The model under review builds one solid part; all positions refer to its coordinate system, in mm. A direction names the side the tool comes from. Round coordinates to 2 decimals unless told otherwise and drop trailing zeros. Order: outer loops, then holes, each group sorted by start corner. A loop starts at its lowest first (then second) coordinate and runs counter-clockwise, first axis right, second up.
```python
from build123d import *

# Parameters (mm, degrees)
SKETCH_1_W          = 50
SKETCH_1_H          = 35
EXTRUDE_1_DEPTH     = 109
SKETCH_2_W          = 50
SKETCH_2_H          = 25
CUT_EXTRUDE_1_DEPTH = 99
CUT_EXTRUDE_2_DEPTH = 11


with BuildPart() as part:
    # 草图1 → 凸台-拉伸1 (new body)
    with BuildSketch(Plane(origin=(0, 0, 0), x_dir=(1, 0, 0), z_dir=(0, 1, 0))):
        Rectangle(SKETCH_1_W, SKETCH_1_H)
    extrude(amount=EXTRUDE_1_DEPTH)

    # 草图2 → 切除-拉伸1 (cut)
    with BuildSketch(Plane(origin=(0, 109, 0), x_dir=(1, 0, 0), z_dir=(0, 1, 0))):
        with Locations((0, 5)):
            Rectangle(SKETCH_2_W, SKETCH_2_H)
    extrude(amount=-CUT_EXTRUDE_1_DEPTH, mode=Mode.SUBTRACT)

    # 草图3 → 切除-拉伸2 (cut, through all)
    with BuildSketch(Plane(origin=(0, 10, 0), x_dir=(1, 0, 0), z_dir=(0, 1, 0))):
        with BuildLine():
            Line((-20.7, 1.5), (-20.7, 9.5))
            ThreePointArc((-20.7, 9.5), (-17.5, 12.7), (-14.3, 9.5))
            Line((-14.3, 9.5), (-14.3, 1.5))
            ThreePointArc((-14.3, 1.5), (-17.5, -1.7), (-20.7, 1.5))
        make_face()
        with BuildLine():
            Line((20.7, 1.5), (20.7, 9.5))
            ThreePointArc((20.7, 9.5), (17.5, 12.7), (14.3, 9.5))
            Line((14.3, 9.5), (14.3, 1.5))
            ThreePointArc((14.3, 1.5), (17.5, -1.7), (20.7, 1.5))
        make_face()
    extrude(amount=-CUT_EXTRUDE_2_DEPTH, mode=Mode.SUBTRACT)


solid = part.part
```
(1) To check wall thickness, follow probe 1 along Z at (x, y) = (-18, 100); probe 2 along Y at (x, z) = (20, 7). State the ranges of each line that lie inside material, in increasing order.
Data:
probe 1: z = 7.5 to 17.5
probe 2: y = 0 to 10
(2) Consider section C-C (x = 6). Write out the cut boundary in (y, z), and give its area (3 significant figures).
Data:
outline: (0, -17.5) - (10, -17.5) - (10, 7.5) - (109, 7.5) - (109, 17.5) - (0, 17.5) - close
area: 1,340 mm2
(3) Consider section A-A (z = -8.5). Write out the cut boundary in (x, y), and give its area (3 significant figures).
Data:
outline: (-25, 0) - (-20.7, 0) - (-20.7, 10) - (-25, 10) - close; (-14.3, 0) - (14.3, 0) - (14.3, 10) - (-14.3, 10) - close; (20.7, 0) - (25, 0) - (25, 10) - (20.7, 10) - close
area: 372 mm2
(4) Consider section D-D (y = 102). Write out the cut boundary in (x, z), and give its area (3 significant figures).
Data:
outline: (-25, 7.5) - (25, 7.5) - (25, 17.5) - (-25, 17.5) - close
area: 500 mm2
(5) For faces 1 (the flat face through (0, 5, -17.5)), 2 (the flat face through (0, 10, -5)), 3 (the flat face through (-20.7, 5, -5)), list the 3-axis set-ups (+Z, -Z, +X, -X, +Y, -Y) from which the entire face can be reached by the end or side of a thin tool; tool diameter is ignored.
Data:
face 1: -Z, +X, -X, +Y, -Y
face 2: -Z, +X, -X, +Y
face 3: +Y, -Y
(6) Draft analysis for pull direction Z (two halves, no side actions). For faces 4 (the flat face through (14.3, 5, -6)), 5 (the flat face through (0, 60, 7.5)), 6 (the flat face through (25, 42, 8)), state which applies: pulls with the +Z half, pulls with the -Z half, needs draft (parallel to the pull), parting line crosses it, or undercut.
Data:
face 4: undercut
face 5: pulls with the -Z half
face 6: needs draft
(7) Consider section B-B (x = 17.5). Write out the cut boundary in (y, z).
Data:
outline: (0, -17.5) - (10, -17.5) - (10, -12.7) - (0, -12.7) - close; (0, 1.7) - (10, 1.7) - (10, 7.5) - (109, 7.5) - (109, 17.5) - (0, 17.5) - close
